from build123d import *

# Parameters (mm, degrees)
SKETCH1_R           = 1.5
BOSS_EXTRUDE1_DEPTH = 4
FILLET1_R           = 0.5
CHAMFER1_SIZE       = 0.2


with BuildPart() as part:
    # Sketch1 → Boss-Extrude1 (new body, symmetric)
    with BuildSketch(Plane(origin=(0, 0, 0), x_dir=(0, -1, 0), z_dir=(1, 0, 0))):
        Circle(SKETCH1_R)
    extrude(amount=BOSS_EXTRUDE1_DEPTH, both=True)

    # Fillet1
    fillet1_edges = [part.edges().sort_by_distance(p)[0] for p in [
        (4, 1.5, 0),
    ]]
    fillet(fillet1_edges, radius=FILLET1_R)

    # Chamfer1
    chamfer1_edges = [part.edges().sort_by_distance(p)[0] for p in [
        (-4, 1.5, 0),
    ]]
    chamfer(chamfer1_edges, length=CHAMFER1_SIZE)


solid = part.part
For this review, take the finished solid that the model builds, in its own axes (mm). Round coordinates to 2 decimals unless told otherwise and drop trailing zeros. Loops run counter-clockwise (first coordinate to the right, second up) from the corner with the lowest first, then second, coordinate; pieces in that order, holes last. Notation, with made-up numbers: (-16, 2.25) - (-5, 2.25) arc R27 ccw to (-5, 26.25) - close; hole circle Ø1 at (26, 87). An arc over 180 degrees is marked (long way). Put each result on its own line as item: value. Start each with the question number.
1. Consider section A-A on x = 2.25. State the section outline as (y, z) points, plus the area to 3 significant figures.
2. Insertion check: P1, Ø1, axis at x = 0, y = -1, coming from the -Z side. The pin has a flat end and moves straight along its axis. Give the tip position at first contact, or say it passes through.
3. Mouldability with a two-part tool opening along X and no side actions: class faces 1 (the flat face through (4, 0, 0)), 2 (the cylindrical face through (-0.1, 1.5, -0.07)), 3 (the flat face through (-4, 0, 0)) as +X half, -X half, draft (parallel to the pull), parting line (faces both ways), or undercut.
4. For probe 1 along Y at (x, z) = (2.5, 0.75); probe 2 along Z at (x, y) = (-1.5, -0.2); probe 3 along Z at (x, y) = (-1, 0.65), list the stretches that pass through material, from the lowest coordinate up. Write a range as [from, to].
Result sheet:
1. outline: circle Ø3 at (0, 0)
1. area: 7.07 mm^2
2. P1: z = -1.41
3. face 1: +X half
3. face 2: draft
3. face 3: -X half
4. probe 1: [-1.3, 1.3]
4. probe 2: [-1.49, 1.49]
4. probe 3: [-1.35, 1.35]
